Build history of the part. All positions in model axes, mm. A direction names the side the tool comes from. Round coordinates to 2 decimals unless told otherwise and drop trailing zeros. Write each loop counter-clockwise with the first axis right and the second up, starting at its lowest first coordinate (ties: lowest second). Pieces come first, ordered by that corner, then holes. Notation, with made-up numbers: M 46,4.5 L 85,4.5 A26 cw 85,38.5 Z; hole C 43.25,52 d7. An arc over 180 degrees is marked long. Use a Markdown table: item, result.
Solid Edge part; units mm, degrees
sketch "Sketch1" plane through (0, 0, 0) normal (0, 0, 1) x (1, 0, 0)
  circle A0 centre (0, 0) radius 31.5
extrude "Protrusion1" add sketch "Sketch1" along normal blind 10
sketch "Sketch2" plane through (0, 0, 0) normal (0, 0, -1) x (1, 0, 0)
  circle A0 centre (0, 0) radius 2
extrude "Extrusionsausschnitt_1" cut sketch "Sketch2" against normal blind 5
sketch "Sketch3" plane through (0, 0, 10) normal (0, 0, 1) x (0, 1, 0)
  line L0 (-21, -19.9) -> (21, -19.9)
  line L1 (21, -19.9) -> (21, 19.9)
  line L2 (21, 19.9) -> (-21, 19.9)
  line L3 (-21, 19.9) -> (-21, -19.9)
extrude "Extrusionsausschnitt_2" cut sketch "Sketch3" against normal blind 2
properties material "Nylon, allgemein"
Q1. Cut at B-B on x = 0. Give the cut face in (y, z), and give its area (3 significant figures).
Response values:
| item | result |
|---|---|
| outline | M -31.5,0 L -2,0 L -2,5 L 2,5 L 2,0 L 31.5,0 L 31.5,10 L 21,10 L 21,8 L -21,8 L -21,10 L -31.5,10 Z |
| area | 526 mm2 |
Q2. Cut at C-C on z = 1.75. Give the cut face in (x, y).
Response values:
| item | result |
|---|---|
| outline | C 0,0 d63; hole C 0,0 d4 |
Q3. Two-plate mould, pull along X, no slides. Class faces 4 (the flat face through (21, 0, 10)), 5 (the cylindrical face through (-4.101, -31.232, 4.93)), 6 (the flat face through (-19.9, 0, 9)): +X half, -X half, draft (parallel to the pull), parting line (faces both ways), or undercut.
Response values:
| item | result |
|---|---|
| face 4 | draft |
| face 5 | parting line |
| face 6 | undercut |
Q4. Drop flat-ended pins along their axis: P1, Ø10, axis at x = -8, y = -19.5, coming from the -Z side; P2, Ø1.5, axis at y = 20.5, z = 4, coming from the +X side; P3, Ø8, axis at x = 15, y = -5, coming from the +Z side; P4, Ø1.6, axis at y = -6.5, z = 9.5, coming from the +X side. Give the stop position or say it passes through.
Response values:
| item | result |
|---|---|
| P1 | stops at z = 0 |
| P2 | stops at x = 24.54 |
| P3 | stops at z = 8 |
| P4 | stops at x = 30.98 |
Q5. Which spindle directions (+Z, -Z, +X, -X, +Y, -Y) get a long thin tool onto all of the face, cutting with end or side? Do faces 1 (the flat face through (7, 0, 0)), 2 (the flat face through (0, 0, 5)), 3 (the flat face through (19.9, 0, 9)). Say none if no direction does.
Response values:
| item | result |
|---|---|
| face 1 | -Z, +X, -X, +Y, -Y |
| face 2 | -Z |
| face 3 | +Z |
Q6. Drill centre lines: L1, parallel to Y at x = 0, z = 3.2; L2, parallel to Z at x = -0.5, y = 10.5; L3, parallel to X at y = -2, z = 9. Where is each one in solid material? Low to high.
Response values:
| item | result |
|---|---|
| L1 | y = -31.5 to -2, 2 to 31.5 |
| L2 | z = 0 to 8 |
| L3 | x = -31.44 to -19.9, 19.9 to 31.44 |
Q7. Cut at D-D on z = 6.75. Give the cut face in (x, y), and give its area (3 significant figures).
Response values:
| item | result |
|---|---|
| outline | C 0,0 d63 |
| area | 3,120 mm2 |
Q8. Cut at A-A on y = 0. Give the cut face in (x, z), and give its area (3 significant figures).
Response values:
| item | result |
|---|---|
| outline | M -31.5,0 L -2,0 L -2,5 L 2,5 L 2,0 L 31.5,0 L 31.5,10 L 19.9,10 L 19.9,8 L -19.9,8 L -19.9,10 L -31.5,10 Z |
| area | 530 mm2 |
